Verification items for the finished model (mm, model axes). Give positions to 0.01 mm unless a question says otherwise; leave off trailing zeros. Write each loop counter-clockwise with the first axis right and the second up, starting at its lowest first coordinate (ties: lowest second). Pieces come first, ordered by that corner, then holes. Notation, with made-up numbers: M 34.5,-4 L 46.5,-4 A34 cw 46.5,34 Z; hole C 50.25,-37 d8. An arc over 180 degrees is marked long. Write item = value, one per line.
from build123d import *

# Parameters (mm, degrees)
SKETCH1_W           = 139.40028
SKETCH1_H           = 152.4
BOSS_EXTRUDE1_DEPTH = 6.35
SKETCH2_W           = 6.35
SKETCH2_H           = 152.4
CUT_EXTRUDE1_DEPTH  = 3.47472
SKETCH3_R           = 8.255
CUT_EXTRUDE2_DEPTH  = 7.35


with BuildPart() as part:
    # Sketch1 → Boss-Extrude1 (new body)
    with BuildSketch(Plane(origin=(0, 0, 0), x_dir=(1, 0, 0), z_dir=(0, 1, 0))):
        with Locations((69.70014, 76.2)):
            Rectangle(SKETCH1_W, SKETCH1_H)
    extrude(amount=BOSS_EXTRUDE1_DEPTH)

    # Sketch2 → Cut-Extrude1 (cut)
    with BuildSketch(Plane(origin=(0, 6.35, 0), x_dir=(1, 0, 0), z_dir=(0, 1, 0))):
        with Locations((3.175, 76.2)):
            Rectangle(SKETCH2_W, SKETCH2_H)
        with Locations((136.22528, 76.2)):
            Rectangle(SKETCH2_W, SKETCH2_H)
    extrude(amount=-CUT_EXTRUDE1_DEPTH, mode=Mode.SUBTRACT)

    # Sketch3 → Cut-Extrude2 (cut, through all)
    with BuildSketch(Plane(origin=(0, 6.35, 0), x_dir=(1, 0, 0), z_dir=(0, 1, 0))):
        with Locations((33.274, 15.408402902)):
            Circle(SKETCH3_R)
    extrude(amount=-CUT_EXTRUDE2_DEPTH, mode=Mode.SUBTRACT)


solid = part.part
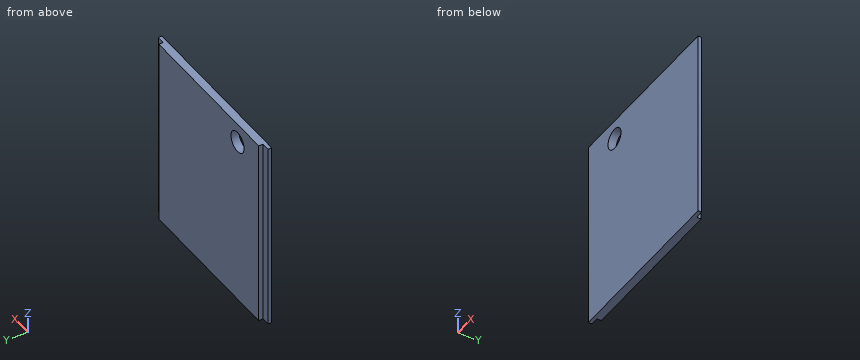
1) Depth check by flat-ended pin: P1, Ø1.9, axis at x = 3, z = -106.5, coming from the +Y side; P2, Ø1, axis at y = 4.5, z = -78.5, coming from the -X side; P3, Ø1, axis at y = 4, z = -105.5, coming from the +X side. Enter the tip coordinate at first touch or a pass-through.
From the geometry:
P1 = 2.88
P2 = 6.35
P3 = 133.05
2) Material ranges on probe 1 along X at (y, z) = (6.25, -25); probe 2 along X at (y, z) = (1, -14.5), recorded low to high. Write a range as from..to.
From the geometry:
probe_1 = 6.35..133.05
probe_2 = 0..25.07, 41.48..139.4
3) Cross-section at B-B on x = 29. Record the boundary of the cut face in (y, z), plus the area to 3 significant figures.
From the geometry:
outline = M 0,-152.4 L 6.35,-152.4 L 6.35,-22.47 L 0,-22.47 Z; M 0,-8.35 L 6.35,-8.35 L 6.35,0 L 0,0 Z
area = 878 mm^2
4) Cross-section at C-C on y = 4. Record the boundary of the cut face in (x, z) (3 decimals).
From the geometry:
outline = M 6.35,-152.4 L 133.05,-152.4 L 133.05,0 L 6.35,0 Z; hole C 33.274,-15.408 d16.51
5) Cross-section at A-A on z = -128.5. Record the boundary of the cut face in (x, y), plus the area to 3 significant figures.
From the geometry:
outline = M 0,0 L 139.4,0 L 139.4,2.88 L 133.05,2.88 L 133.05,6.35 L 6.35,6.35 L 6.35,2.88 L 0,2.88 Z
area = 841 mm^2
